Verification items for this drawing (mm, ordinates from the low corner). Give positions to 0.01 mm unless a question says otherwise; leave off trailing zeros. Loops run counter-clockwise (first coordinate to the right, second up) from the corner with the lowest first, then second, coordinate; pieces in that order, holes last. Notation, with made-up numbers: (5, -34) -> (10, -34) arc R26 cw to (10, 4) -> close; hole circle Ø8 at (36, 2.5). An arc over 180 degrees is marked (long way). Write each question's results on one line, items separated by ' | '. Start each with the question number.
1) Depth check by flat-ended pin: pin 1 (9.5 mm diameter, centred on x = 34.925, z = 9.525, fed in from -Y); pin 2 (6.5 mm diameter, centred on x = 60.325, z = 9.525, fed in from +Y). Enter the tip coordinate at first touch or a pass-through.
2) Scan line: line 1 (Z direction, x = 38, y = 3.25). Record every from-to range of solid material in increasing order. Write a range as from..to.
3) Draft check along Z on the marked faces 1, 2, 3 and 4. Enter one of: pulls with the +Z half, pulls with the -Z half, needs draft (parallel to the pull), parting line crosses it, or undercut.
4) Sectioned sample at B-B on y = 7. Count the separate pieces of the cut face and the enclosed holes in it, then the cut area to 3 significant figures.
5) Sectioned sample at A-A on x = 60.5. Record the cut outline in (y, z).
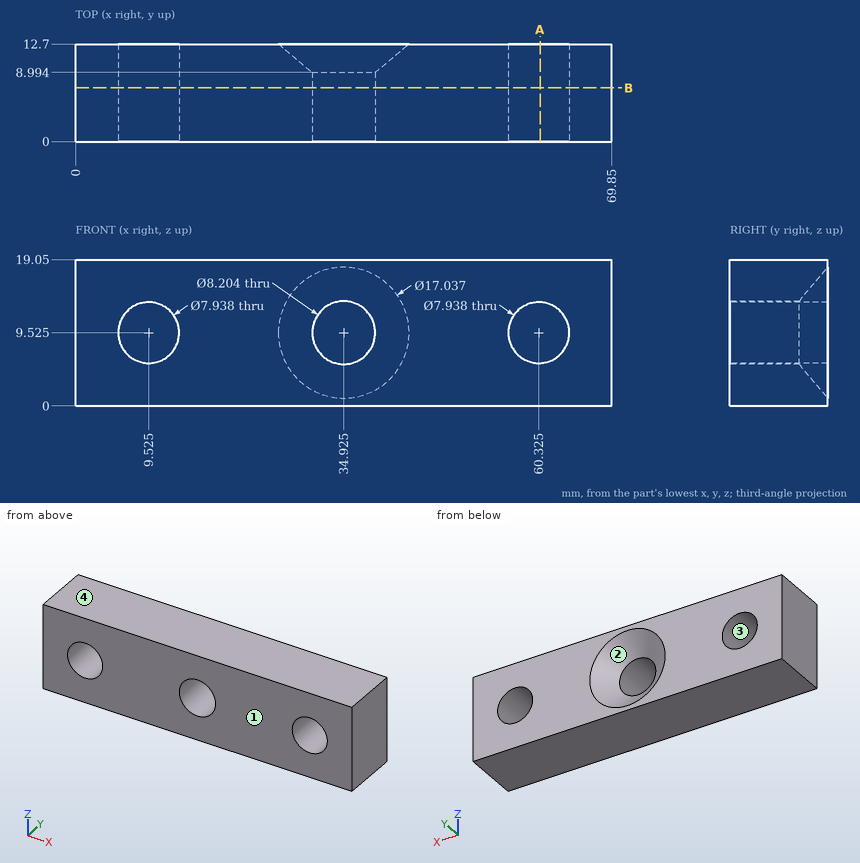
Result:
1) pin 1: y = 0 | pin 2: through
2) line 1: 0..6.81, 12.24..19.05
3) face 1: needs draft | face 2: undercut | face 3: undercut | face 4: pulls with the +Z half
4) separate pieces: 1 | enclosed holes: 3 | area: 1,180 mm^2
5) outline: (0, 0) -> (12.7, 0) -> (12.7, 5.56) -> (0, 5.56) -> close; (0, 13.49) -> (12.7, 13.49) -> (12.7, 19.05) -> (0, 19.05) -> close
